The listing builds one solid part. Answer for the finished solid, in the listing's coordinates (mm). Face numbers are marked on the shaded views. A direction names the side the tool comes from. Give positions to 0.01 mm unless a question says otherwise; leave off trailing zeros. Write each loop counter-clockwise with the first axis right and the second up, starting at its lowest first coordinate (ties: lowest second). Pieces come first, ordered by that corner, then holes. Notation, with made-up numbers: M -22.5,25 L 29.5,25 A21 ccw 29.5,62 Z; hole C -6,71.5 d10. An arc over 180 degrees is marked long. Return JSON: item names as keys, results as strings.
from build123d import *

# Parameters (mm, degrees)
BOSS_EXTRUDE1_DEPTH       = 10.95
F_6_CLEARANCE_HOLE1_D     = 3.7973
F_6_32_TAPPED_HOLE1_D     = 2.7051
F_6_32_TAPPED_HOLE1_DEPTH = 9.398
F_6_32_TAPPED_HOLE1_TIP   = 0.81269403


with BuildPart() as part:
    # Sketch1 → Boss-Extrude1 (new body)
    with BuildSketch(Plane.XY):
        Polygon((-20.955, 22.701840042), (-14.605, 22.701840042), (-14.605, 0), (14.605, 0), (14.605, 22.701840042), (20.955, 22.701840042), (20.955, -6.35), (-20.955, -6.35), align=None)
    extrude(amount=BOSS_EXTRUDE1_DEPTH)

    # #6 Clearance Hole1 (through all)
    with Locations(Plane(origin=(0, -6.35, 0), x_dir=(-1, 0, 0), z_dir=(0, -1, 0))):
        with Locations((-6.985, -5.475), (6.985, -5.475)):
            Hole(F_6_CLEARANCE_HOLE1_D / 2)

    # #6-32 Tapped Hole1
    with Locations(Plane(origin=(0, 22.701840042, 0), x_dir=(1, 0, 0), z_dir=(0, 1, 0))):
        with Locations((17.653, -5.475), (-17.653, -5.475)):
            Hole(F_6_32_TAPPED_HOLE1_D / 2, depth=F_6_32_TAPPED_HOLE1_DEPTH)
            with Locations((0, 0, -(F_6_32_TAPPED_HOLE1_DEPTH + F_6_32_TAPPED_HOLE1_TIP / 2))):  # 118° drill point
                Cone(0, F_6_32_TAPPED_HOLE1_D / 2, F_6_32_TAPPED_HOLE1_TIP, mode=Mode.SUBTRACT)


solid = part.part
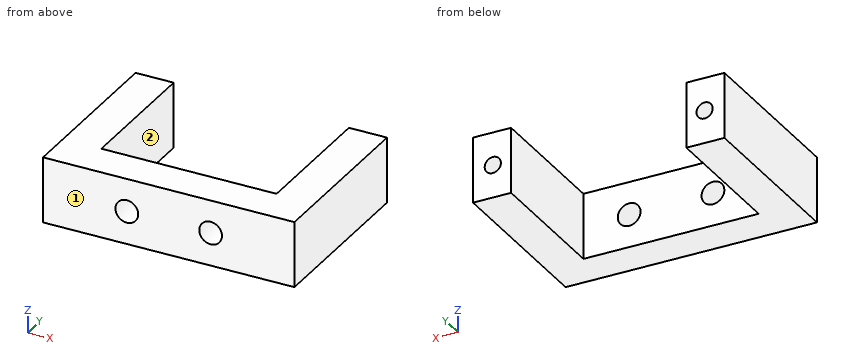
Item 1: A cutting plane is placed at C-C, the plane z = 8. Write down the section's boundary in (x, y) (3 decimals), plus the area to 3 significant figures.
Geometry results:
{"outline": "M -20.955,-6.35 L 20.955,-6.35 L 20.955,22.702 L 14.605,22.702 L 14.605,0 L -14.605,0 L -14.605,22.702 L -20.955,22.702 Z", "area": "554 mm2"}
Item 2: A cutting plane is placed at D-D, the plane x = 6.5. Write down the section's boundary in (y, z).
Geometry results:
{"outline": "M -6.35,0 L 0,0 L 0,3.64 L -6.35,3.64 Z; M -6.35,7.31 L 0,7.31 L 0,10.95 L -6.35,10.95 Z"}
Item 3: A cutting plane is placed at B-B, the plane y = 20.5. Write down the section's boundary in (x, z) (3 decimals), plus the area to 3 significant figures.
Geometry results:
{"outline": "M -20.955,0 L -14.605,0 L -14.605,10.95 L -20.955,10.95 Z; M 14.605,0 L 20.955,0 L 20.955,10.95 L 14.605,10.95 Z; hole C -17.653,5.475 d2.705; hole C 17.653,5.475 d2.705", "area": "128 mm2"}
Item 4: Given pin 1 Ø3.5 at (x, z) = (-0.5, 6) entering from +Y, flat-ended and moving along its own axis, determine where the tip first touches the part or whether it passes through.
Geometry results:
{"pin 1": "stops at y = 0"}
Item 5: Find the intervals of material crossed by line 1 (X direction, y = 1.25, z = 4) (3 decimals); line 2 (Y direction, x = 13.5, z = 4.25); line 3 (X direction, y = -1.25, z = 7) (3 decimals), in increasing order.
Geometry results:
{"line 1": "x = -20.955 to -14.605, 14.605 to 20.955", "line 2": "y = -6.35 to 0", "line 3": "x = -20.955 to -8.116, -5.854 to 5.854, 8.116 to 20.955"}
Item 6: A cutting plane is placed at A-A, the plane y = 3.75. Write down the section's boundary in (x, z) (3 decimals), plus the area to 3 significant figures.
Geometry results:
{"outline": "M -20.955,0 L -14.605,0 L -14.605,10.95 L -20.955,10.95 Z; M 14.605,0 L 20.955,0 L 20.955,10.95 L 14.605,10.95 Z", "area": "139 mm2"}
Item 7: Which of the six approach directions +Z, -Z, +X, -X, +Y, -Y give full straight-line access (tool end or side, diameter ignored) to the marked faces 1 and 2?
Geometry results:
{"face 1": "+Z, -Z, +X, -X, -Y", "face 2": "+Z, -Z, +Y"}
